Verification items for the finished model (mm, model axes). A direction names the side the tool comes from. Coordinates: 2 decimals unless noted, no trailing zeros. Order: outer loops, then holes, each group sorted by start corner. A loop starts at its lowest first (then second) coordinate and runs counter-clockwise, first axis right, second up. Notation, with made-up numbers: M -18.75,85.25 L 38.25,85.25 A12 cw 38.25,106.25 Z; hole C 48,2 d6. An arc over 180 degrees is marked long. Write item = value, one per line.
```python
from build123d import *

# Parameters (mm, degrees)
SKETCH2_W           = 51.895920804
SKETCH2_H           = 8.246585089
BOSS_EXTRUDE1_DEPTH = 49
SKETCH3_W           = 40.788974389
SKETCH3_H           = 8.246585089
CUT_EXTRUDE1_DEPTH  = 30
SKETCH4_W           = 22.869815576
SKETCH4_H           = 16.619980412
CUT_EXTRUDE2_DEPTH  = 6
SKETCH5_W           = 27.5
SKETCH5_H           = 4
CUT_EXTRUDE3_DEPTH  = 2.5
SKETCH12_W          = 27.5
SKETCH12_H          = 4
CUT_EXTRUDE6_DEPTH  = 2.5
SKETCH15_W          = 45.788974389
SKETCH15_H          = 4
CUT_EXTRUDE7_DEPTH  = 17.5
SKETCH17_W          = 7.778908367
SKETCH17_H          = 4.284963324
BOSS_EXTRUDE2_DEPTH = 10.5
SKETCH18_R          = 1.5
CUT_EXTRUDE8_DEPTH  = 5


with BuildPart() as part:
    # Sketch2 → Boss-Extrude1 (new body)
    with BuildSketch(Plane.XY):
        with Locations((-27.854725768, 12.114483507)):
            Rectangle(SKETCH2_W, SKETCH2_H)
    extrude(amount=BOSS_EXTRUDE1_DEPTH)

    # Sketch3 → Cut-Extrude1 (cut)
    with BuildSketch(Plane(origin=(0, 0, 0), x_dir=(-1, 0, 0), z_dir=(0, 0, -1))):
        with Locations((27.921471274, 12.114483507)):
            Rectangle(SKETCH3_W, SKETCH3_H)
    extrude(amount=-CUT_EXTRUDE1_DEPTH, mode=Mode.SUBTRACT)

    # Sketch4 → Cut-Extrude2 (cut)
    with BuildSketch(Plane(origin=(0, 16.237776051, 0), x_dir=(1, 0, 0), z_dir=(0, 1, 0))):
        with Locations((-34.588870015, -38.97443395)):
            Rectangle(SKETCH4_W, SKETCH4_H)
    extrude(amount=-CUT_EXTRUDE2_DEPTH, mode=Mode.SUBTRACT)

    # Sketch5 → Cut-Extrude3 (cut)
    with BuildSketch(Plane.ZY.offset(7.52698408)):
        with Locations((16.25, 10.791190962)):
            Rectangle(SKETCH5_W, SKETCH5_H)
    extrude(amount=-CUT_EXTRUDE3_DEPTH, mode=Mode.SUBTRACT)

    # Sketch12 → Cut-Extrude6 (cut)
    with BuildSketch(Plane(origin=(-48.315958469, 0, 0), x_dir=(0, 0, -1), z_dir=(1, 0, 0))):
        with Locations((-16.25, 10.791190962)):
            Rectangle(SKETCH12_W, SKETCH12_H)
    extrude(amount=-CUT_EXTRUDE6_DEPTH, mode=Mode.SUBTRACT)

    # Sketch15 → Cut-Extrude7 (cut)
    with BuildSketch(Plane(origin=(0, 0, 30), x_dir=(-1, 0, 0), z_dir=(0, 0, -1))):
        with Locations((27.921471274, 10.791190962)):
            Rectangle(SKETCH15_W, SKETCH15_H)
    extrude(amount=-CUT_EXTRUDE7_DEPTH, mode=Mode.SUBTRACT)

    # Sketch17 → Boss-Extrude2 (add)
    with BuildSketch(Plane(origin=(0, 16.237776051, 0), x_dir=(1, 0, 0), z_dir=(0, 1, 0))):
        with Locations((-49.913231987, -33.995977251)):
            Rectangle(SKETCH17_W, SKETCH17_H)
    extrude(amount=BOSS_EXTRUDE2_DEPTH)

    # Sketch18 → Cut-Extrude8 (cut)
    with BuildSketch(Plane.XY.offset(36.138458913)):
        with Locations((-50.239621596, 23.429782287)):
            Circle(SKETCH18_R)
    extrude(amount=-CUT_EXTRUDE8_DEPTH, mode=Mode.SUBTRACT)


solid = part.part
```
Item 1: Sectioned sample at A-A, the plane z = 6. Enter the section's corners in (x, y).
Report:
outline = M -53.8,7.99 L -48.32,7.99 L -48.32,8.79 L -50.82,8.79 L -50.82,12.79 L -48.32,12.79 L -48.32,16.24 L -53.8,16.24 Z; M -7.53,7.99 L -1.91,7.99 L -1.91,16.24 L -7.53,16.24 L -7.53,12.79 L -5.03,12.79 L -5.03,8.79 L -7.53,8.79 Z
Item 2: Tool access check on faces 4 (the flat face through (-50, 21, 31.853)), 5 (the flat face through (-50, 21, 36.138)), 6 (the flat face through (-35, 15, 47.284)), 7 (the flat face through (-48.316, 13, 15)). Record the directions out of +Z, -Z, +X, -X, +Y, -Y that give a thin tool (end or side, any length) a straight path to the whole face; none if there is none.
Report:
face_4 = -Z, +X, -X, +Y
face_5 = +Z, +X, -X, +Y
face_6 = +Y
face_7 = -Z, +Y, -Y
Item 3: Sectioned sample at D-D, the plane z = 42.5. Enter the section's corners in (x, y).
Report:
outline = M -53.8,7.99 L -1.91,7.99 L -1.91,16.24 L -23.15,16.24 L -23.15,12.79 L -5.03,12.79 L -5.03,8.79 L -50.82,8.79 L -50.82,12.79 L -46.02,12.79 L -46.02,16.24 L -53.8,16.24 Z
Item 4: Release check for a two-part mould opening along Y. For faces 1 (the flat face through (-50.816, 11, 25)), 2 (the flat face through (-7.527, 13, 15)), 3 (the flat face through (-50, 26.738, 34)) record: pulls with the +Y half, pulls with the -Y half, needs draft (parallel to the pull), parting line crosses it, or undercut.
Report:
face_1 = undercut
face_2 = needs draft
face_3 = pulls with the +Y half
Item 5: Sectioned sample at B-B, the plane x = -35. Enter the section's corners in (y, z).
Report:
outline = M 7.99,30 L 8.79,30 L 8.79,47.5 L 12.79,47.5 L 12.79,47.28 L 16.24,47.28 L 16.24,49 L 7.99,49 Z; M 12.79,30 L 16.24,30 L 16.24,30.66 L 12.79,30.66 Z
Item 6: Scan lines: L1, parallel to X at y = 13.75, z = 23; L2, parallel to X at y = 9.75, z = 24.5; L3, parallel to Y at x = -11, z = 40.5. Record each from-to range of solid material in increasing order. Write a range as from..to.
Report:
L1 = -53.8..-48.32, -7.53..-1.91
L2 = -53.8..-50.82, -5.03..-1.91
L3 = 7.99..8.79, 12.79..16.24
Item 7: Gauge pin test, flat ends, axial feed: pin 1 (8 mm diameter, centred on y = 21, z = 6.5, fed in from +X); pin 2 (6 mm diameter, centred on x = -48.5, y = 23.5, fed in from -Z); pin 3 (1 mm diameter, centred on x = -39, y = 15, fed in from -Z). Record the tip position at first contact, or that the pin passes through.
Report:
pin_1 = through
pin_2 = 31.85
pin_3 = 30
Item 8: Sectioned sample at C-C, the plane y = 15.5. Enter the section's corners in (x, z), then the cut area to 3 significant figures.
Report:
outline = M -53.8,0 L -48.32,0 L -48.32,30 L -7.53,30 L -7.53,0 L -1.91,0 L -1.91,49 L -53.8,49 Z; hole M -46.02,30.66 L -23.15,30.66 L -23.15,47.28 L -46.02,47.28 Z
area = 939 mm^2
